Design review of the part built by this model. Coordinates are the model's own, in mm. Give positions to 0.01 mm unless a question says otherwise; leave off trailing zeros. Write each loop counter-clockwise with the first axis right and the second up, starting at its lowest first coordinate (ties: lowest second). Pieces come first, ordered by that corner, then holes. Notation, with made-up numbers: (21, 75.5) -> (49, 75.5) arc R14 ccw to (49, 81.5) -> close; hole circle Ø9 at (1.5, -24.75). An arc over 180 degrees is marked (long way). Answer as a JSON object with one key per item and string values.
```python
from build123d import *

# Parameters (mm, degrees)
SKETCH_R   = 4
SKETCH_R_2 = 4.05
SKETCH_R_3 = 2.5
PAD_DEPTH  = 4


with BuildPart() as part:
    # Sketch → Pad (new body)
    with BuildSketch(Plane.XZ):
        with BuildLine():
            Line((-134.93, 13.165085), (-134.93, 20.165085))
            ThreePointArc((-129.93, 25.165085), (-133.465534, 23.700619), (-134.93, 20.165085))
            Line((-129.93, 25.165085), (130.07, 25.165085))
            ThreePointArc((135.07, 20.165085), (133.605534, 23.700619), (130.07, 25.165085))
            Line((135.07, 20.165085), (135.07, 10.165085))
            ThreePointArc((130.07, 5.165085), (133.605534, 6.629551), (135.07, 10.165085))
            Line((130.07, 5.165085), (130.023889, 5.165085))
            ThreePointArc((110.116111, 5.165085), (120.07, 1.093085), (130.023889, 5.165085))
            Line((110.116111, 5.165085), (48.852111, 5.165085))
            ThreePointArc((48.852111, 5.165085), (30.534511, 0.724409), (16.284037, -11.611638))
            ThreePointArc((-18.547693, -7.482184), (-2.354598, -19.860913), (16.284037, -11.611638))
            ThreePointArc((-18.547693, -7.482184), (-27.746929, 3.887274), (-41.732309, 8.165085))
            Line((-129.93, 8.165085), (-41.732309, 8.165085))
            ThreePointArc((-134.93, 13.165085), (-133.465534, 9.629551), (-129.93, 8.165085))
        make_face()
        Circle(SKETCH_R, mode=Mode.SUBTRACT)
        with Locations((120.07, 15.295085)):
            Circle(SKETCH_R_2, mode=Mode.SUBTRACT)
        with Locations((-122.93, 16.665085)):
            Circle(SKETCH_R_3, mode=Mode.SUBTRACT)
        with Locations((-47.93, 16.665085)):
            Circle(SKETCH_R_3, mode=Mode.SUBTRACT)
    extrude(amount=PAD_DEPTH)


solid = part.part
```
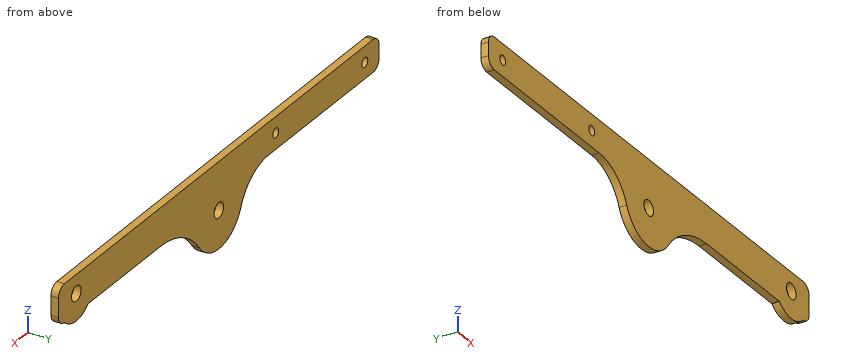
(1) Clearance check with flat-ended pins moving along their axes: pin 1 (1 mm diameter, centred on x = 106.5, y = -1.5, fed in from -Z); pin 2 (1.5 mm diameter, centred on y = -3.5, z = -2, fed in from +X). State where each tip first meets the part, or that it passes through.
Here are the results:
{"pin 1": "stops at z = 5.17", "pin 2": "stops at x = 27.13"}
(2) We need section B-B, the plane y = -0.9. State the section outline as (x, z) points, then the cut area to 3 significant figures.
Here are the results:
{"outline": "(-134.93, 13.17) arc R5 ccw to (-129.93, 8.17) -> (-41.73, 8.17) arc R25 cw to (-18.55, -7.48) arc R20 ccw to (16.28, -11.61) arc R40 cw to (48.85, 5.17) -> (110.12, 5.17) arc R14.2 ccw to (130.02, 5.17) -> (130.07, 5.17) arc R5 ccw to (135.07, 10.17) -> (135.07, 20.17) arc R5 ccw to (130.07, 25.17) -> (-129.93, 25.17) arc R5 ccw to (-134.93, 20.17) -> close; hole circle Ø5 at (-122.93, 16.67); hole circle Ø5 at (-47.93, 16.67); hole circle Ø8 at (0, 0); hole circle Ø8.1 at (120.07, 15.3)", "area": "5,980 mm²"}
(3) We need section D-D, the plane x = -61. State the section outline as (y, z) points, then the cut area to 3 significant figures.
Here are the results:
{"outline": "(-4, 8.17) -> (0, 8.17) -> (0, 25.17) -> (-4, 25.17) -> close", "area": "68.0 mm²"}
(4) For line 1 along Z through (x, y) = (-47.93, -0.9); line 2 along X through (y, z) = (-2.25, 17); line 3 along Z through (x, y) = (-96, -3.35), list the stretches that pass through material, from the lowest coordinate up.
Here are the results:
{"line 1": "z = 8.17 to 14.17, 19.17 to 25.17", "line 2": "x = -134.93 to -125.41, -120.45 to -50.41, -45.45 to 116.4, 123.74 to 135.07", "line 3": "z = 8.17 to 25.17"}
(5) We need section A-A, the plane x = 0. State the section outline as (y, z) points.
Here are the results:
{"outline": "(-4, -20) -> (0, -20) -> (0, -4) -> (-4, -4) -> close; (-4, 4) -> (0, 4) -> (0, 25.17) -> (-4, 25.17) -> close"}
(6) We need section C-C, the plane x = 120.07. State the section outline as (y, z) points, then the cut area to 3 significant figures.
Here are the results:
{"outline": "(-4, 1.09) -> (0, 1.09) -> (0, 11.25) -> (-4, 11.25) -> close; (-4, 19.35) -> (0, 19.35) -> (0, 25.17) -> (-4, 25.17) -> close", "area": "63.9 mm²"}
